Here's the drawing with two shaded views (mm, measured from the low corner). I have some questions. A direction names the side the tool comes from. Give positions to 0.01 mm unless a question says otherwise; leave off trailing zeros. Loops run counter-clockwise (first coordinate to the right, second up) from the corner with the lowest first, then second, coordinate; pieces in that order, holes last. Notation, with made-up numbers: M -37.75,6.5 L -19.75,6.5 A16 ccw -19.75,15.5 Z; hole C -23.75,-15.5 d7. An arc over 180 degrees is marked long. Put each result on its own line as item: value. Start each with the question number.
1) If we mould it in two halves opening along Z, with no side actions, what happens to the marked faces 1, 2 and 3? For each: +Z half, -Z half, draft (parallel to the pull), parting line (faces both ways), or undercut.
2) Please list where these lines run through material, in increasing order: line 1 along Z through (x, y) = (3.5, 34.5); line 2 along X through (y, z) = (39.5, 32) (3 decimals); line 3 along Y through (x, z) = (13.5, 21) (3 decimals). Write a range as from..to.
3) Imagine slicing it at A-A (y = 22). Write out the boundary of the cut face in (x, z) (3 decimals), then the cut area to 3 significant figures.
4) For the marked faces 4 and 5, which set-ups out of +Z, -Z, +X, -X, +Y, -Y let a thin tool reach every point of the face, with its end or its side?
5) For P1, Ø1.5, axis at x = 9, y = 20, coming from the +Z side; P2, Ø1, axis at y = 6.5, z = 29.5, coming from the -X side; P3, Ø4, axis at x = 21.5, z = 29.5, coming from the -Y side, each with a flat end and sliding along its axis, tell me the tip position at first contact or that it passes through.
6) Imagine slicing it at B-B (x = 23.25). Write out the boundary of the cut face in (y, z) (3 decimals).
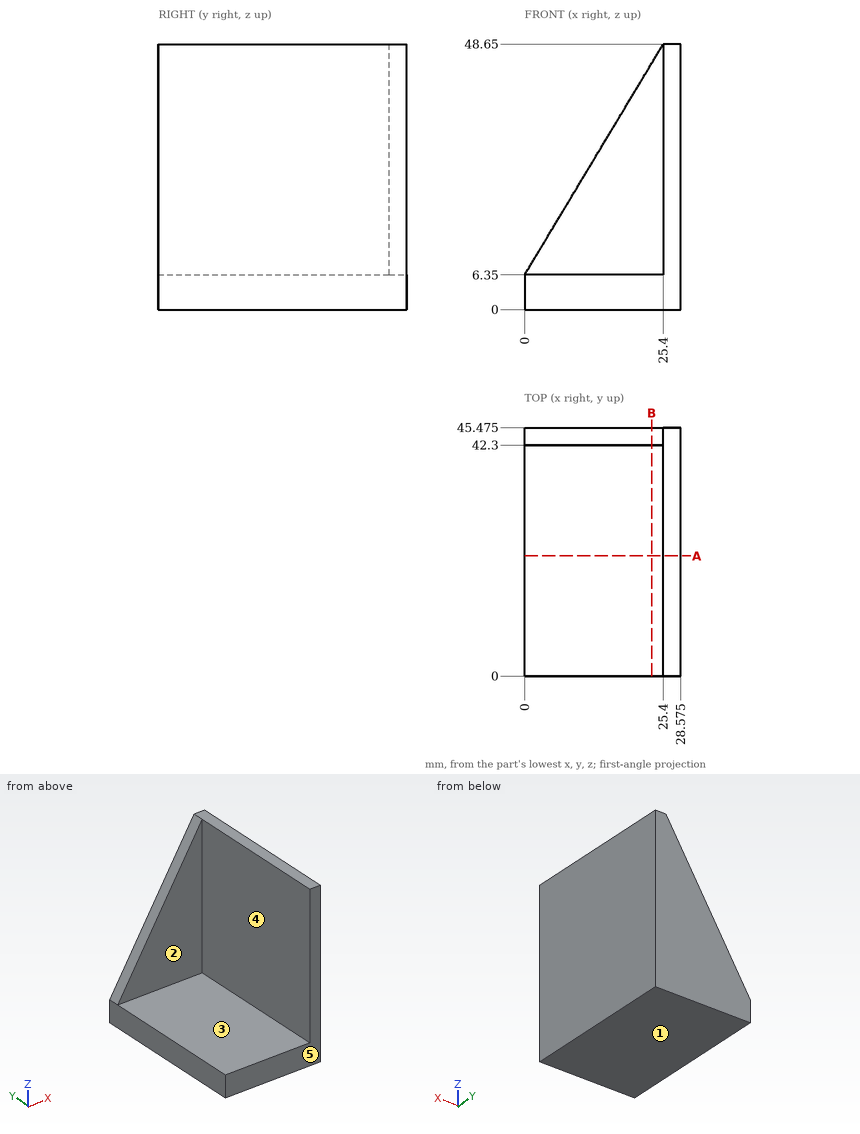
Recorded:
1. face 1: -Z half
1. face 2: draft
1. face 3: +Z half
2. line 1: 0..6.35
2. line 2: 25.4..28.575
2. line 3: 42.3..45.475
3. outline: M 0,0 L 28.575,0 L 28.575,48.65 L 25.4,48.65 L 25.4,6.35 L 0,6.35 Z
3. area: 316 mm²
4. face 4: +Z, -X, -Y
4. face 5: +Z, -Z, +X, -X, -Y
5. P1: z = 6.35
5. P2: x = 25.4
5. P3: y = 42.3
6. outline: M 0,0 L 45.475,0 L 45.475,45.069 L 42.3,45.069 L 42.3,6.35 L 0,6.35 Z
